Verification items for the finished model (mm, model axes). A direction names the side the tool comes from. Give positions to 0.01 mm unless a question says otherwise; leave off trailing zeros. Order: outer loops, then holes, each group sorted by start corner. A loop starts at its lowest first (then second) coordinate and runs counter-clockwise, first axis right, second up.
from build123d import *

# Parameters (mm, degrees)
F1_DEPTH      = 5
F1_DEPTH_BACK = 5
F3_DEPTH      = 2
F5_W          = 9
F5_H          = 5.5
F6_DEPTH      = 25
F7_SIZE       = 1.99999


# Not quite as in the source:
# - a fillet or chamfer is up to 0.001 mm smaller than in the source, because OpenCascade refuses the exact size


with BuildPart() as f1:
    # F0 (on Front) → F1 (new body, two sides)
    with BuildSketch(Plane.XZ) as f1_sk:
        with BuildLine():
            Line((8, 0), (12.5, 0))
            ThreePointArc((12.5, 0), (0, 12.5), (-12.5, 0))
            Line((-12.5, 0), (-8, 0))
            ThreePointArc((-8, 0), (0, 8), (8, 0))
        make_face()
        Polygon((26, 0), (12.5, 0), (8, 0), (8, -10), (26, -10), align=None)
        Polygon((-8, 0), (-12.5, 0), (-26, 0), (-26, -10), (-8, -10), align=None)
    extrude(amount=F1_DEPTH)
    extrude(f1_sk.sketch, amount=-F1_DEPTH_BACK)

    # F2 (on face) → F3 (join)
    with BuildSketch(Plane(origin=(0, 5, 0), x_dir=(-1, 0, 0), z_dir=(0, 1, 0))):
        with BuildLine():
            Line((6, 0), (8, 0))
            ThreePointArc((8, 0), (0, 8), (-8, 0))
            Line((-8, 0), (-6, 0))
            ThreePointArc((-6, 0), (0, 6), (6, 0))
        make_face()
    extrude(amount=-F3_DEPTH)

    # F4: F1 across plane


with BuildPart() as f1_1:
    add(f1.part)
    add(f1.part.mirror(Plane.XZ))

    # F5 (on face) → F6 (cut)
    with BuildSketch(Plane.XY):
        with Locations((-17, 0)):
            Rectangle(F5_W, F5_H)
        with Locations((17, 0)):
            Rectangle(F5_W, F5_H)
    extrude(amount=-F6_DEPTH, mode=Mode.SUBTRACT)

    # F7 (size 2 in the source; OpenCascade refuses exactly that, so slightly less here)
    f7_edges = [f1_1.edges().sort_by_distance(p)[0] for p in [
        (-8, -4, 0),
        (-8, 0, 0),
        (-8, 4, 0),
        (8, 0, 0),
        (8, -4, 0),
        (8, 4, 0),
    ]]
    chamfer(f7_edges, length=F7_SIZE)


solid = f1_1.part
(1) Section check B-B, the plane x = 20.5. Enter the section's corners in (y, z).
Solved:
outline: (-5, -10) - (-2.75, -10) - (-2.75, 0) - (-5, 0) - close; (2.75, -10) - (5, -10) - (5, 0) - (2.75, 0) - close
(2) Scan lines: line 1 (X direction, y = 1, z = -3); line 2 (Y direction, x = 4.5, z = 6); line 3 (Y direction, x = -14, z = -6.75). Record each from-to range of solid material in increasing order.
Solved:
line 1: x = -26 to -21.5, -12.5 to -8, 8 to 12.5, 21.5 to 26
line 2: y = -5 to -3, 3 to 5
line 3: y = -5 to -2.75, 2.75 to 5
(3) Go/stop test with flat-tipped pins: pin 1 (3 mm diameter, centred on x = -1.5, z = 4, fed in from -Y); pin 2 (5 mm diameter, centred on x = -20.5, y = 2.5, fed in from +Z); pin 3 (5 mm diameter, centred on y = -3.5, z = 8.5, fed in from -X); pin 4 (2 mm diameter, centred on y = -1.5, z = 3, fed in from -X). Record where each tip stops, or that it passes through.
Solved:
pin 1: passes through
pin 2: stops at z = 0
pin 3: stops at x = -10.97
pin 4: stops at x = -12.34
(4) Section check C-C, the plane y = -1.5. Enter the section's corners in (x, z).
Solved:
outline: (-26, -10) - (-21.5, -10) - (-21.5, 0) - (-26, 0) - close; (-12.5, -10) - (-8, -10) - (-8, 0) arc R8 cw to (8, 0) - (8, -10) - (12.5, -10) - (12.5, 0) arc R12.5 ccw to (-12.5, 0) - close; (21.5, -10) - (26, -10) - (26, 0) - (21.5, 0) - close
(5) Set-up check for faces 4 (the flat face through (-12.5, 0, -5)), 5 (the flat face through (22, 0, 0)), 6 (the flat face through (-7, -4, -1)), 7 (the flat face through (-8, 0, -5)): record each of +Z, -Z, +X, -X, +Y, -Y from which the full face is reachable in a straight line by a thin tool's end or side.
Solved:
face 4: +Z, -Z
face 5: +Z, +X, +Y, -Y
face 6: -Z, +Y, -Y
face 7: -Z
(6) Release check for a two-part mould opening along Y. For faces 1 (the cylindrical face through (0, 0, 8)), 2 (the cylindrical face through (0, -4, 6)), 3 (the flat face through (6.1, -5, 1.4)) record: pulls with the +Y half, pulls with the -Y half, needs draft (parallel to the pull), parting line crosses it, or undercut.
Solved:
face 1: undercut
face 2: needs draft
face 3: pulls with the -Y half
(7) Section check A-A, the plane z = -5.5. Enter the section's corners in (x, y), then the cut area to 3 significant figures.
Solved:
outline: (-26, -5) - (-8, -5) - (-8, 5) - (-26, 5) - close; (8, -5) - (26, -5) - (26, 5) - (8, 5) - close; hole (-21.5, -2.75) - (-12.5, -2.75) - (-12.5, 2.75) - (-21.5, 2.75) - close; hole (12.5, -2.75) - (21.5, -2.75) - (21.5, 2.75) - (12.5, 2.75) - close
area: 261 mm2
